Geometry: final body of the model. Coordinates: model frame, mm. Round coordinates to 2 decimals unless told otherwise and drop trailing zeros. Use CSV: the item, a comma, the result in double quotes.
Autodesk Inventor part; units mm, degrees
ref_plane "YZ Plane" through (0, 0, 0) normal (1, 0, 0) x (0, 1, 0)
ref_plane "XZ Plane" through (0, 0, 0) normal (0, 1, 0) x (-1, 0, 0)
ref_plane "XY Plane" through (0, 0, 0) normal (0, 0, 1) x (1, 0, 0)
sketch "Sketch1" plane through (0, 0, 0) normal (0, 0, 1) x (1, 0, 0)
  line L0 (0, 0) -> (20, 0)
  line L1 (20, 0) -> (20, 17.5)
  line L2 (20, 17.5) -> (0, 17.5)
  line L3 (0, 17.5) -> (0, 0)
  dimension "d0" = 20
  dimension "d1" = 17.5
extrude "Extrusion1" add sketch "Sketch1" along normal blind 800
sketch "Sketch2" plane through (0, 17.5, 0) normal (0, 1, 0) x (1, 0, 0)
  circle A0 centre (10, -20) radius 3
  line L0 (20, 0) -> (0, 0)
  point P0 (10, 0)
  dimension "d4" = 6
  dimension "d5" = 20
extrude "Extrusion2" cut sketch "Sketch2" against normal up to surface (17.5 mm away)
sketch "Sketch3" plane through (0, 17.5, 0) normal (0, 1, 0) x (1, 0, 0)
  circle A0 centre (10, -20) radius 4.75
  circle A1 centre (10, -20) radius 3 construction
  point P0 (0, 0)
  dimension "d8" = 9.5
extrude "Extrusion3" cut sketch "Sketch3" against normal blind 8.5
pattern_linear "Rectangular Pattern1" count 18 spacing 60 along (0, 0, 1) of "Extrusion2", "Extrusion3"
properties part number "HGW20CC_Rail_800mm_ACTUAL"
Item 1: Material intervals for line 1 (X direction, y = 12, z = 260); line 2 (X direction, y = 6, z = 440); line 3 (Y direction, x = 12, z = 262.5), sorted ascending.
Final values:
line 1,"x = 0 to 5.25, 14.75 to 20"
line 2,"x = 0 to 7, 13 to 20"
line 3,"y = 0 to 9"
Item 2: Pin query (flat end, axial travel): P1, Ø3, axis at x = 12.5, z = 78.5, coming from the +Y side. Return the tip coordinate at first contact, or that it passes through.
Final values:
P1,"stops at y = 9"
Item 3: Mould query, pull axis Y, two halves, no side actions, for faces 1 (the flat face through (10, 17.5, 394)), 2 (the flat face through (0, 9, 394)), 3 (the flat face through (10, 0, 394)). Classes: released by +Y, released by -Y, zero draft, split by the parting line, or undercut.
Final values:
face 1,"released by +Y"
face 2,"zero draft"
face 3,"released by -Y"
Item 4: Section A-A on y = 4.75. Give the number of separate pieces and of enclosed holes in the cut face, plus the area to 3 significant figures.
Final values:
separate pieces,"1"
enclosed holes,"13"
area,"15,600 mm²"
